```python
from build123d import *

# Parameters (mm, degrees)
ESQUISSE1_R                = 35
BOSS_EXTRU_1_DEPTH         = 40
ESQUISSE6_W                = 70
ESQUISSE6_H                = 40
BOSS_EXTRU_3_DEPTH         = 70
ESQUISSE2_R                = 30
ENL_V_MAT_EXTRU_1_DEPTH    = 40
BOSS_EXTRU_2_START         = 40
BOSS_EXTRU_2_DEPTH         = 40
ESQUISSE4_W                = 4
ESQUISSE4_H                = 20
ENL_V_MAT_EXTRU_2_DEPTH    = 40
ESQUISSE5_W                = 2.5
ESQUISSE5_H                = 5
ENL_V_MAT_EXTRU_3_DEPTH    = 91.44888059
R_P_TITION_LIN_AIRE1_COUNT = 4
R_P_TITION_LIN_AIRE1_PITCH = 10
ENL_V_MAT_EXTRU_4_DEPTH    = 107.77078252
ESQUISSE8_W                = 70
ESQUISSE8_H                = 55
BOSS_EXTRU_4_DEPTH         = 5
D_GAGEMENT_M51_D           = 5.5
CONG_1_R                   = 30
CONG_2_R                   = 5


with BuildPart() as part:
    # Esquisse1 → Boss.-Extru.1 (new body)
    with BuildSketch(Plane.XY):
        Circle(ESQUISSE1_R)
    extrude(amount=BOSS_EXTRU_1_DEPTH)

    # Esquisse6 → Boss.-Extru.3 (add)
    with BuildSketch(Plane(origin=(0, 0, 0), x_dir=(1, 0, 0), z_dir=(0, 1, 0))):
        with Locations((0, -20)):
            Rectangle(ESQUISSE6_W, ESQUISSE6_H)
    extrude(amount=-BOSS_EXTRU_3_DEPTH)

    # Esquisse2 → Enlèv. mat.-Extru.1 (cut)
    with BuildSketch(Plane.XY.offset(40)):
        Circle(ESQUISSE2_R)
    extrude(amount=-ENL_V_MAT_EXTRU_1_DEPTH, mode=Mode.SUBTRACT)

    # Esquisse3 → Boss.-Extru.2 (add)
    with BuildSketch(Plane.XY.offset(BOSS_EXTRU_2_START)):
        with BuildLine():
            Line((-6, 29.393876913), (-6, 48.393876913))
            Line((-6, 48.393876913), (6, 48.393876913))
            Line((6, 48.393876913), (6, 29.393876913))
            ThreePointArc((6, 29.393876913), (0, 30), (-6, 29.393876913))
        make_face()
    extrude(amount=-BOSS_EXTRU_2_DEPTH)

    # Esquisse4 → Enlèv. mat.-Extru.2 (cut)
    with BuildSketch(Plane.XY.offset(40)):
        with Locations((0, 38.393876913)):
            Rectangle(ESQUISSE4_W, ESQUISSE4_H)
    extrude(amount=-ENL_V_MAT_EXTRU_2_DEPTH, mode=Mode.SUBTRACT)

    # Esquisse5 → Enlèv. mat.-Extru.3 (cut, through all)
    with BuildSketch(Plane(origin=(6, 0, 0), x_dir=(0, 0, -1), z_dir=(1, 0, 0))):
        with Locations((-34.75, 41.893876913)):
            Rectangle(ESQUISSE5_W, ESQUISSE5_H)
    enl_v_mat_extru_3 = extrude(amount=-ENL_V_MAT_EXTRU_3_DEPTH, mode=Mode.SUBTRACT)

    # Répétition linéaire1: Enlèv. mat.-Extru.3 ×4
    with Locations(*[(0, 0, -i * R_P_TITION_LIN_AIRE1_PITCH) for i in range(1, R_P_TITION_LIN_AIRE1_COUNT)]):
        add(enl_v_mat_extru_3, mode=Mode.SUBTRACT)

    # Esquisse7 → Enlèv. mat.-Extru.4 (cut, through all)
    with BuildSketch(Plane.ZY.offset(35)):
        Polygon((-15, -70), (20, -35), (55, -70), align=None)
    extrude(amount=-ENL_V_MAT_EXTRU_4_DEPTH, mode=Mode.SUBTRACT)

    # Esquisse8 → Boss.-Extru.4 (add)
    with BuildSketch(Plane(origin=(0, -7.5, -7.5), x_dir=(1, 0, 0), z_dir=(0, -0.7071067811865515, -0.7071067811865436))):
        with Locations((0, 66.390872965)):
            Rectangle(ESQUISSE8_W, ESQUISSE8_H)
    extrude(amount=-BOSS_EXTRU_4_DEPTH)

    # Dégagement M51 (through all)
    with Locations(Plane(origin=(0, -3.964466094, -3.964466094), x_dir=(1, 0, 0), z_dir=(0, 0.7071067811865517, 0.7071067811865435))):
        with Locations((-25, -78.890872965), (25, -78.890872965)):
            Hole(D_GAGEMENT_M51_D / 2)

    # Congé1
    cong_1_edges = [part.edges().sort_by_distance(p)[0] for p in [
        (0, -47.928932188, 40),
    ]]
    fillet(cong_1_edges, radius=CONG_1_R)

    # Congé2
    cong_2_edges = [part.edges().sort_by_distance(p)[0] for p in [
        (4, 48.393876913, 40),
        (4, 48.393876913, 0),
        (-4, 48.393876913, 0),
        (-4, 48.393876913, 40),
    ]]
    fillet(cong_2_edges, radius=CONG_2_R)


solid = part.part
```
Verification items for the finished model (mm, model axes). A direction names the side the tool comes from. Coordinates: 2 decimals unless noted, no trailing zeros. Order: outer loops, then holes, each group sorted by start corner. A loop starts at its lowest first (then second) coordinate and runs counter-clockwise, first axis right, second up. Notation, with made-up numbers: (-21.5, -19) - (-12.5, -19) arc R13 cw to (-12.5, 1) - close; hole circle Ø4 at (-8, 7). An arc over 180 degrees is marked (long way). Return JSON: item names as keys, results as strings.
(1) Access from +Z, -Z, +X, -X, +Y, -Y to the whole of each face (thin tool, end or side, straight path). Record for faces 1 (the flat face through (2, 39, 20)), 2 (the cylindrical face through (27.01, 22.26, 19.72)), 3 (the flat face through (-0.49, -72.15, 60.63)), 4 (the flat face through (-4, 39.394, 5)), 5 (the flat face through (-6, 41, 20)).
Filled sheet:
{"face 1": "+Z, -Z, +Y", "face 2": "+Z, -Z, +X, +Y", "face 3": "+Z, +X, -X, -Y", "face 4": "+X, -X", "face 5": "+Z, -Z, -X, +Y"}
(2) Section check D-D, the plane x = 0. Record the cut outline in (y, z).
Filled sheet:
{"outline": "(-73.89, 58.89) - (-35, 20) - (-55, 0) - (-30, 0) - (-30, 40) - (-35.5, 40) arc R30 cw to (-56.72, 48.79) - (-70.36, 62.43) - close"}
(3) Section check A-A, the plane y = 7. Record the cut outline in (x, z), and give its area (3 significant figures).
Filled sheet:
{"outline": "(-34.29, 0) - (-29.17, 0) - (-29.17, 40) - (-34.29, 40) - close; (29.17, 0) - (34.29, 0) - (34.29, 40) - (29.17, 40) - close", "area": "410 mm^2"}
(4) Mould release check, pull along Z, two halves, no side actions. Record for faces 6 (the flat face through (0, -38, 0)), 7 (the cylindrical face through (-22.253, -61.456, 49.942)), 8 (the flat face through (0, -31, 40)), 9 (the flat face through (-4, 39.394, 15)): pulls with the +Z half, pulls with the -Z half, needs draft (parallel to the pull), parting line crosses it, or undercut.
Filled sheet:
{"face 6": "pulls with the -Z half", "face 7": "undercut", "face 8": "pulls with the +Z half", "face 9": "undercut"}
(5) Thickness scan on line 1 along X through (y, z) = (0, 8); line 2 along Y through (x, z) = (-23, 6.5); line 3 along Z through (x, y) = (-16, 28). Record the ranges inside material, lowest first.
Filled sheet:
{"line 1": "x = -35 to -30, 30 to 35", "line 2": "y = -48.5 to -19.26, 19.26 to 26.38", "line 3": "z = 0 to 40"}
(6) Section check B-B, the plane x = -19. Record the cut outline in (y, z).
Filled sheet:
{"outline": "(-73.89, 58.89) - (-35, 20) - (-55, 0) - (-23.22, 0) - (-23.22, 40) - (-35.5, 40) arc R30 cw to (-56.72, 48.79) - (-70.36, 62.43) - close; (23.22, 0) - (29.39, 0) - (29.39, 40) - (23.22, 40) - close"}
(7) Section check C-C, the plane z = 29. Record the cut outline in (x, y), and give its area (3 significant figures).
Filled sheet:
{"outline": "(-35, -44) - (35, -44) - (35, 0) arc R35 ccw to (6, 34.48) - (6, 48.39) - (2, 48.39) - (2, 29.93) arc R30 cw (long way) to (-2, 29.93) - (-2, 48.39) - (-6, 48.39) - (-6, 34.48) arc R35 ccw to (-35, 0) - close", "area": "2,270 mm^2"}
(8) Go/stop test with flat-tipped pins: pin 1 (1.2 mm diameter, centred on x = -4, z = 34.5, fed in from -Y); pin 2 (12 mm diameter, centred on x = 25, z = 11.5, fed in from +Y); pin 3 (1.2 mm diameter, centred on x = -4, y = 42.5, fed in from +Z). Record where each tip stops, or that it passes through.
Filled sheet:
{"pin 1": "stops at y = -50.1", "pin 2": "stops at y = 29.39", "pin 3": "stops at z = 40"}
